Check sheet for the modelled part. Datum: model origin and axes. Units: mm. A direction names the side the tool comes from. Give positions to 0.01 mm unless a question says otherwise; leave off trailing zeros. Loops run counter-clockwise (first coordinate to the right, second up) from the corner with the lowest first, then second, coordinate; pieces in that order, holes last. Notation, with made-up numbers: M 8,-16.5 L 60,-16.5 A22 ccw 60,5.5 Z; hole C -3.75,57 d2. An arc over 180 degrees is marked long. Put each result on its own line as item: value. Start each with the question number.
```python
from build123d import *

# Parameters (mm, degrees)
SKETCH_1_R      = 44.5
SKETCH_1_R_2    = 42.5
EXTRUDE_7_DEPTH = 1


with BuildPart() as part:
    # Эскиз1 → Бобышка-Вытянуть7 (new body)
    # profile 1 of 9: a face of its own
    with BuildSketch(Plane(origin=(0, 0, 0), x_dir=(1, 0, 0), z_dir=(0, 1, 0))):
        with Locations(Location((0, 0, 0), (0, 0, 270))):
            Circle(SKETCH_1_R)
        Circle(SKETCH_1_R_2, mode=Mode.SUBTRACT)
    # profile 2 of 9: a face of its own
    with BuildSketch(Plane(origin=(0, 0, 0), x_dir=(1, 0, 0), z_dir=(0, 1, 0))):
        with BuildLine():
            Line((-35.470093763, 1), (-42.488233665, 1))
            ThreePointArc((-42.488233665, 1), (-42.5, 0), (-42.488233665, -1))
            Line((-42.488233665, -1), (-34.537478446, -1))
            Line((-34.537478446, -1), (-6.690761703, 32.186424721))
            Line((-6.690761703, 32.186424721), (-2.450567073, 8.139086006))
            ThreePointArc((-2.450567073, 8.139086006), (-1.47600951, 8.370865901), (-0.480951567, 8.486382362))
            Line((-0.480951567, 8.486382362), (-5.465925634, 36.75757516))
            Line((-5.465925634, 36.75757516), (-35.470093763, 1))
        make_face()
    # profile 3 of 9: a face of its own
    with BuildSketch(Plane(origin=(0, 0, 0), x_dir=(1, 0, 0), z_dir=(0, 1, 0))):
        with BuildLine():
            ThreePointArc((8.5, 0), (5.837889673, 6.17811008), (-0.480951567, 8.486382362))
            Line((-0.480951567, 8.486382362), (-0.130467861, 6.498690494))
            ThreePointArc((-0.130467861, 6.498690494), (4.549832904, 4.64209226), (6.5, 0))
            ThreePointArc((6.5, 0), (5.28680158, -3.781498255), (2.100083368, -6.151394139))
            Line((2.100083368, -6.151394139), (2.450567073, -8.139086006))
            ThreePointArc((2.450567073, -8.139086006), (6.822016568, -5.070511802), (8.5, 0))
        make_face()
    # profile 4 of 9: a face of its own
    with BuildSketch(Plane(origin=(0, 0, 0), x_dir=(1, 0, 0), z_dir=(0, 1, 0))):
        with BuildLine():
            Line((-0.130467861, 6.498690494), (-0.480951567, 8.486382362))
            ThreePointArc((-0.480951567, 8.486382362), (-1.47600951, 8.370865901), (-2.450567073, 8.139086006))
            Line((-2.450567073, 8.139086006), (-2.100083368, 6.151394139))
            ThreePointArc((-2.100083368, 6.151394139), (-1.128713155, 6.401250395), (-0.130467861, 6.498690494))
        make_face()
    # profile 5 of 9: a face of its own
    with BuildSketch(Plane(origin=(0, 0, 0), x_dir=(1, 0, 0), z_dir=(0, 1, 0))):
        with BuildLine():
            ThreePointArc((0.480951567, -8.486382362), (1.47600951, -8.370865901), (2.450567073, -8.139086006))
            Line((2.450567073, -8.139086006), (2.100083368, -6.151394139))
            ThreePointArc((2.100083368, -6.151394139), (1.128713155, -6.401250395), (0.130467861, -6.498690494))
            Line((0.130467861, -6.498690494), (0.480951567, -8.486382362))
        make_face()
    # profile 6 of 9: a face of its own
    with BuildSketch(Plane(origin=(0, 0, 0), x_dir=(1, 0, 0), z_dir=(0, 1, 0))):
        with BuildLine():
            Line((-2.100083368, 6.151394139), (-2.450567073, 8.139086006))
            ThreePointArc((-2.450567073, 8.139086006), (-8.370865901, -1.47600951), (0.480951567, -8.486382362))
            Line((0.480951567, -8.486382362), (0.130467861, -6.498690494))
            ThreePointArc((0.130467861, -6.498690494), (-6.401250395, -1.128713155), (-2.100083368, 6.151394139))
        make_face()
    # profile 7 of 9: a face of its own
    with BuildSketch(Plane(origin=(0, 0, 0), x_dir=(1, 0, 0), z_dir=(0, 1, 0))):
        with BuildLine():
            ThreePointArc((42.5, 0), (42.497058315, 0.50003461), (42.488233665, 1))
            Line((42.488233665, 1), (34.537478446, 1))
            Line((34.537478446, 1), (6.690761703, -32.186424721))
            Line((6.690761703, -32.186424721), (2.450567073, -8.139086006))
            ThreePointArc((2.450567073, -8.139086006), (1.47600951, -8.370865901), (0.480951567, -8.486382362))
            Line((0.480951567, -8.486382362), (5.465925634, -36.75757516))
            Line((5.465925634, -36.75757516), (35.470093763, -1))
            Line((35.470093763, -1), (42.488233665, -1))
            ThreePointArc((42.488233665, -1), (42.497058315, -0.50003461), (42.5, 0))
        make_face()
    # profile 8 of 9: a face of its own
    with BuildSketch(Plane(origin=(0, 0, 0), x_dir=(1, 0, 0), z_dir=(0, 1, 0))):
        with BuildLine():
            Line((-0.130467861, 6.498690494), (-0.480951567, 8.486382362))
            ThreePointArc((-0.480951567, 8.486382362), (-1.47600951, 8.370865901), (-2.450567073, 8.139086006))
            Line((-2.450567073, 8.139086006), (-2.100083368, 6.151394139))
            ThreePointArc((-2.100083368, 6.151394139), (-1.128713155, 6.401250395), (-0.130467861, 6.498690494))
        make_face()
    # profile 9 of 9: a face of its own
    with BuildSketch(Plane(origin=(0, 0, 0), x_dir=(1, 0, 0), z_dir=(0, 1, 0))):
        with BuildLine():
            ThreePointArc((0.480951567, -8.486382362), (1.47600951, -8.370865901), (2.450567073, -8.139086006))
            Line((2.450567073, -8.139086006), (2.100083368, -6.151394139))
            ThreePointArc((2.100083368, -6.151394139), (1.128713155, -6.401250395), (0.130467861, -6.498690494))
            Line((0.130467861, -6.498690494), (0.480951567, -8.486382362))
        make_face()
    extrude(amount=EXTRUDE_7_DEPTH)


solid = part.part
```
Q1. Thickness scan on line 1 along X through (y, z) = (0.9, 24); line 2 along X through (y, z) = (0.1, -31.5); line 3 along Z through (x, y) = (-38.5, 0.6). Record the ranges inside material, lowest first. Write a range as [from, to].
Q2. Section check D-D, the plane z = 3.5. Record the cut outline in (x, y), then the cut area to 3 significant figures.
Q3. Access from +Z, -Z, +X, -X, +Y, -Y to the whole of each face (thin tool, end or side, straight path). Record for faces 4 (the face through (2.939, 0.493, 22.424)), 5 (the face through (-4, 1, 6)).
Q4. Section check B-B, the plane z = 23. Record the cut outline in (x, y).
Q5. Section check C-C, the plane x = -38. Record the cut outline in (y, z).
Q6. Depth check by flat-ended pin: P1, Ø0.5, axis at x = 39.5, y = 0.5, coming from the -Z side; P2, Ø12, axis at x = -32, z = 23, coming from the -Y side. Enter the tip coordinate at first touch or a pass-through.
Q7. Mould release check, pull along Z, two halves, no side actions. Record for faces 1 (the face through (30.075, 0.493, -32.798)), 2 (the face through (20.81, 0.49, 15.36)), 3 (the face through (-4, 0, 6)): pulls with the +Z half, pulls with the -Z half, needs draft (parallel to the pull), parting line crosses it, or undercut.
Found:
1. line 1: x = [-37.47, -35.07], [3.22, 5.25], [13.56, 16.17], [35.07, 37.47]
1. line 2: x = [-31.43, -28.53], [-9.88, -7.27], [-6.57, -4.54], [28.53, 31.43]
1. line 3: z = [-22.32, -18], [-1, 1], [18, 22.32]
2. outline: M -44.36,0 L -42.36,0 L -42.36,1 L -44.36,1 Z; M -7.75,0 L -5.48,0 L -5.48,1 L -7.75,1 Z; M 5.48,0 L 7.75,0 L 7.75,1 L 5.48,1 Z; M 30.76,0 L 33.37,0 L 33.37,1 L 30.76,1 Z; M 42.36,0 L 44.36,0 L 44.36,1 L 42.36,1 Z
2. area: 11.2 mm^2
3. face 4: +Y, -Y
3. face 5: +Z, -Z, +X, -X, +Y
4. outline: M -38.1,0 L -35.74,0 L -35.74,1 L -38.1,1 Z; M 3.04,0 L 5.07,0 L 5.07,1 L 3.04,1 Z; M 14.4,0 L 17.01,0 L 17.01,1 L 14.4,1 Z; M 35.74,0 L 38.1,0 L 38.1,1 L 35.74,1 Z
5. outline: M 0,-23.16 L 1,-23.16 L 1,-19.03 L 0,-19.03 Z; M 0,-1 L 1,-1 L 1,1 L 0,1 Z; M 0,19.03 L 1,19.03 L 1,23.16 L 0,23.16 Z
6. P1: stops at z = -20.97
6. P2: stops at y = 0
7. face 1: parting line crosses it
7. face 2: undercut
7. face 3: needs draft
